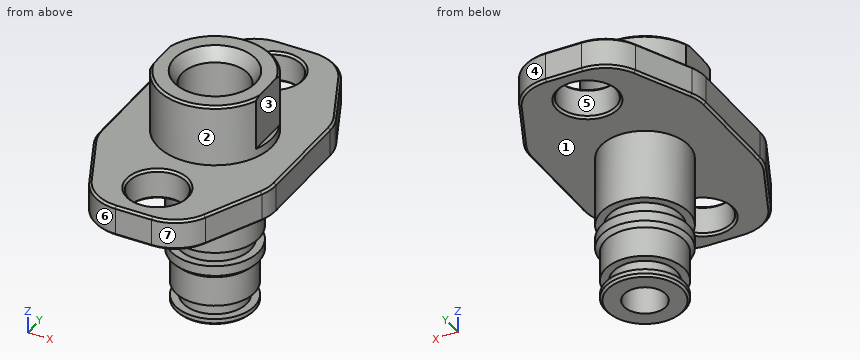
from build123d import *

# Parameters (mm, degrees)
SKETCH2_OUTSIDE_W  = 94.65
SKETCH2_OUTSIDE_H  = 94.65
SKETCH2_OUTSIDE_R  = 6.5
CUT_EXTRUDE1_DEPTH = 21
SKETCH5_W          = 2.091476768
SKETCH5_H          = 18
CUT_EXTRUDE2_DEPTH = 12
CIRPATTERN1_COUNT  = 2
CIRPATTERN1_ANGLE  = 180
CHAMFER1_SIZE      = 0.5


with BuildPart() as part:
    # Sketch1 → Revolve1 (revolve)
    with BuildSketch(Plane(origin=(0, 0, 0), x_dir=(0, 0, -1), z_dir=(1, 0, 0)), mode=Mode.PRIVATE) as revolve1_sk:
        Polygon((14, 35), (21, 35), (21, 9.95), (37, 9.95), (37, 8.15), (40.2, 8.15), (40.2, 9.95), (42.5, 9.95), (43.46, 8.99), (50.3, 8.99), (50.3, 7.2), (53.5, 7.2), (53.5, 8.99), (54.5, 8.99), (55, 8.49), (55, 4.75), (18.652366702, 4.75), (17, 7.5), (3, 7.5), (0, 9.232050808), (0, 12.5), (0.5, 13), (14, 13), align=None)
    revolve(revolve1_sk.sketch.rotate(Axis((0, 0, 0), (0, 0, -1)), 90), axis=Axis((0, 0, 0), (0, 0, -1)))

    # Sketch2 outside → Cut-Extrude1 (cut)
    # profile 1 of 3: a face of its own
    with BuildSketch(Plane.XY):
        Rectangle(SKETCH2_OUTSIDE_W, SKETCH2_OUTSIDE_H)
        with BuildLine():
            Line((-4.112562412, 34), (4.112562412, 34))
            ThreePointArc((4.112562412, 34), (9.495586596, 32.427517466), (13.185668477, 28.204610128))
            Line((13.185668477, 28.204610128), (19.073106065, 15.500139543))
            ThreePointArc((19.073106065, 15.500139543), (19.765527652, 13.448311261), (20, 11.295529415))
            Line((20, 11.295529415), (20, -11.295529415))
            ThreePointArc((20, -11.295529415), (19.765527652, -13.448311261), (19.073106065, -15.500139543))
            Line((19.073106065, -15.500139543), (13.185668477, -28.204610128))
            ThreePointArc((13.185668477, -28.204610128), (9.495586596, -32.427517466), (4.112562412, -34))
            Line((4.112562412, -34), (-4.112562412, -34))
            ThreePointArc((-4.112562412, -34), (-9.495586596, -32.427517466), (-13.185668477, -28.204610128))
            Line((-13.185668477, -28.204610128), (-19.073106065, -15.500139543))
            ThreePointArc((-19.073106065, -15.500139543), (-19.765527652, -13.448311261), (-20, -11.295529415))
            Line((-20, -11.295529415), (-20, 11.295529415))
            ThreePointArc((-20, 11.295529415), (-19.765527652, 13.448311261), (-19.073106065, 15.500139543))
            Line((-19.073106065, 15.500139543), (-13.185668477, 28.204610128))
            ThreePointArc((-13.185668477, 28.204610128), (-9.495586596, 32.427517466), (-4.112562412, 34))
        make_face(mode=Mode.SUBTRACT)
    # profile 2 of 3: a face of its own
    with BuildSketch(Plane.XY):
        with Locations((0, 24)):
            Circle(SKETCH2_OUTSIDE_R)
    # profile 3 of 3: a face of its own
    with BuildSketch(Plane.XY):
        with Locations((0, -24)):
            Circle(SKETCH2_OUTSIDE_R)
    extrude(amount=-CUT_EXTRUDE1_DEPTH, mode=Mode.SUBTRACT)

    # Sketch5 → Cut-Extrude2 (cut)
    with BuildSketch(Plane.XY):
        with Locations((-13.045738384, -0.152764218)):
            Rectangle(SKETCH5_W, SKETCH5_H)
    cut_extrude2 = extrude(amount=-CUT_EXTRUDE2_DEPTH, mode=Mode.SUBTRACT)

    # CirPattern1: Cut-Extrude2 ×2 about axis
    cirpattern1_axis = Axis((0, 0, 0), (0, 0, 1))
    for i in range(1, CIRPATTERN1_COUNT):
        add(cut_extrude2.rotate(cirpattern1_axis, i * CIRPATTERN1_ANGLE / (CIRPATTERN1_COUNT - 1)), mode=Mode.SUBTRACT)

    # Chamfer1
    chamfer1_edges = [part.edges().sort_by_distance(p)[0] for p in [
        (-6.5, 24, -21),
        (-6.5, 24, -14),
        (-6.5, -24, -21),
        (-6.5, -24, -14),
        (20, 0, -21),
        (19.765527652, 13.448311261, -21),
        (16.129387271, 21.852374836, -21),
        (9.495586596, 32.427517466, -21),
        (0, 34, -21),
        (-9.495586596, 32.427517466, -21),
        (-16.129387271, 21.852374836, -21),
        (-19.765527652, 13.448311261, -21),
        (-20, 0, -21),
        (-19.765527652, -13.448311261, -21),
        (-16.129387271, -21.852374836, -21),
        (-9.495586596, -32.427517466, -21),
        (0, -34, -21),
        (9.495586596, -32.427517466, -21),
        (16.129387271, -21.852374836, -21),
        (19.765527652, -13.448311261, -21),
        (19.765527652, 13.448311261, -14),
        (20, 0, -14),
        (19.765527652, -13.448311261, -14),
        (16.129387271, -21.852374836, -14),
        (9.495586596, -32.427517466, -14),
        (0, -34, -14),
        (-9.495586596, -32.427517466, -14),
        (-16.129387271, -21.852374836, -14),
        (-19.765527652, -13.448311261, -14),
        (-20, 0, -14),
        (-19.765527652, 13.448311261, -14),
        (-16.129387271, 21.852374836, -14),
        (-9.495586596, 32.427517466, -14),
        (0, 34, -14),
        (9.495586596, 32.427517466, -14),
        (16.129387271, 21.852374836, -14),
    ]]
    chamfer(chamfer1_edges, length=CHAMFER1_SIZE)


solid = part.part
Build history of the part. All positions in model axes, mm. Face numbers are marked on the shaded views. A direction names the side the tool comes from. Give positions to 0.01 mm unless a question says otherwise; leave off trailing zeros. Loops run counter-clockwise (first coordinate to the right, second up) from the corner with the lowest first, then second, coordinate; pieces in that order, holes last. Notation, with made-up numbers: (52.25, 0) - (83.25, 0) arc R7 ccw to (83.25, 12) - close; hole circle Ø10 at (73.25, 6). An arc over 180 degrees is marked (long way). Write item = value, one per line. Start each with the question number.
1) Band-saw the part on C-C on x = 0. Count the separate pieces of the cut face and the enclosed holes in it, plus the area to 3 significant figures.
2) Band-saw the part on D-D on z = -22.5. Give the cut face in (x, y), plus the area to 3 significant figures.
3) Tool access for the marked faces 1, 2, 3 and 4: list every direction of +Z, -Z, +X, -X, +Y, -Y with a clear straight run to the whole face (end or side of a thin tool).
4) Probe probe 1 along Y at (x, z) = (0, -19.1); probe 2 along Z at (x, y) = (-10, -20); probe 3 along Y at (x, z) = (0, -9.75). List the from-to ranges inside material, lowest first. Write a range as from..to.
5) Pull direction X, two halves, no side cores. Call the marked faces 5, 6 and 7: +X half, -X half, draft (parallel to the pull), parting line (faces both ways), or undercut.
6) Band-saw the part on B-B on y = -24. Give the cut face in (x, z).
7) Band-saw the part on A-A on z = -9. Give the cut face in (x, y), plus the area to 3 significant figures.
8) Drop flat-ended pins along their axis: pin 1 Ø8 at (y, z) = (2, -3.5) entering from +X; pin 2 Ø1 at (x, z) = (-6, -25.5) entering from -Y; pin 3 Ø0.8 at (x, y) = (12.5, -1.5) entering from +Z. Give the stop position or say it passes through.
Final values:
q1.separate_pieces = 4
q1.enclosed_holes = 0
q1.area = 661 mm²
q2.outline = circle Ø19.9 at (0, 0); hole circle Ø9.5 at (0, 0)
q2.area = 240 mm²
q3.face_1 = -Z
q3.face_2 = +Z
q3.face_3 = +Z, +X, +Y, -Y
q3.face_4 = +Z, -Z, +X, +Y
q4.probe_1 = -34..-30.5, -17.5..-4.75, 4.75..17.5, 30.5..34
q4.probe_2 = -21..-14
q4.probe_3 = -13..-7.5, 7.5..13
q5.face_5 = undercut
q5.face_6 = -X half
q5.face_7 = +X half
q6.outline = (-15.13, -20.5) - (-14.58, -21) - (-7, -21) - (-6.5, -20.5) - (-6.5, -14.5) - (-7, -14) - (-14.58, -14) - (-15.13, -14.5) - close; (6.5, -20.5) - (7, -21) - (14.58, -21) - (15.13, -20.5) - (15.13, -14.5) - (14.58, -14) - (7, -14) - (6.5, -14.5) - close
q7.outline = (-12, -5) arc R13 ccw to (12, -5) - (12, 5) arc R13 ccw to (-12, 5) - close; hole circle Ø15 at (0, 0)
q7.area = 341 mm²
q8.pin_1 = 12
q8.pin_2 = -8.29
q8.pin_3 = -12
